Source: three-view drawing plus pictorial views. Frame: mm from the lowest corner of the part. A direction names the side the tool comes from. Give positions to 0.01 mm unless a question says otherwise; leave off trailing zeros. Loops run counter-clockwise (first coordinate to the right, second up) from the corner with the lowest first, then second, coordinate; pieces in that order, holes last. Notation, with made-up numbers: (61.5, 35.25) - (75.5, 35.25) arc R23 ccw to (75.5, 67.25) - close; hole circle Ø5 at (66, 32.25). An arc over 180 degrees is marked (long way). Answer as a JSON object with one key per item and string values.
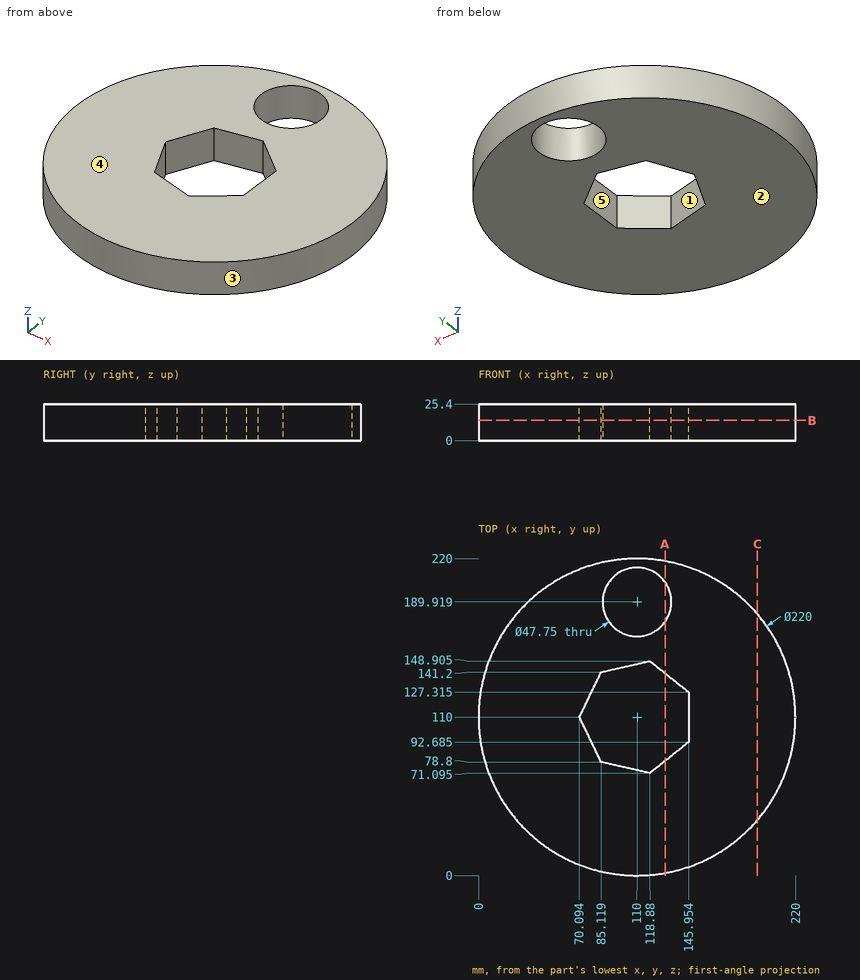
Item 1: Access query for the marked faces 4 and 5. Directions: +Z, -Z, +X, -X, +Y, -Y. A direction counts if a zero-diameter tool reaches every point of the face in a straight line with its end or side. Return the directions, or none.
Geometry check:
{"face 4": "+Z, +X, -X, +Y, -Y", "face 5": "+Z, -Z"}
Item 2: Material intervals for line 1 (Y direction, x = 108, z = 23.5); line 2 (Y direction, x = 110, z = 13); line 3 (X direction, y = 176, z = 18), sorted ascending. Write a range as [from, to].
Geometry check:
{"line 1": "y = [0.02, 73.58], [146.42, 166.13], [213.71, 219.98]", "line 2": "y = [0, 73.12], [146.88, 166.04], [213.79, 220]", "line 3": "x = [22, 90.6], [129.4, 198]"}
Item 3: Cut plane C-C (x = 193.5). Return loops of the section in (y, z), then the cut area to 3 significant figures.
Geometry check:
{"outline": "(38.39, 0) - (181.61, 0) - (181.61, 25.4) - (38.39, 25.4) - close", "area": "3,640 mm2"}
Item 4: Mould query, pull axis X, two halves, no side actions, for the marked faces 1, 2 and 3. Classes: released by +X, released by -X, zero draft, split by the parting line, or undercut.
Geometry check:
{"face 1": "undercut", "face 2": "zero draft", "face 3": "split by the parting line"}
Item 5: Contact query for flat-ended pins moving along their axis: P1, Ø12, axis at y = 52, z = 6.5, coming from the +X side; P2, Ø6, axis at y = 125, z = 12, coming from the +X side; P3, Ø5, axis at x = 68, z = 21.5, coming from the +Y side; P4, Ø1, axis at x = 46, y = 94, coming from the -Z side. Output: stop coordinate, or through.
Geometry check:
{"P1": "stops at x = 206.93", "P2": "stops at x = 219.34", "P3": "stops at y = 212.66", "P4": "stops at z = 0"}
Item 6: Cut plane B-B (z = 14). Give the number of separate pieces and of enclosed holes in the cut face, then the cut area to 3 significant figures.
Geometry check:
{"separate pieces": "1", "enclosed holes": "2", "area": "31,900 mm2"}
Item 7: Cut plane A-A (x = 129.5). Return loops of the section in (y, z).
Geometry check:
{"outline": "(1.74, 0) - (79.56, 0) - (79.56, 25.4) - (1.74, 25.4) - close; (140.44, 0) - (176.14, 0) - (176.14, 25.4) - (140.44, 25.4) - close; (203.69, 0) - (218.26, 0) - (218.26, 25.4) - (203.69, 25.4) - close"}
